Check sheet for the modelled part. Datum: model origin and axes. Units: mm. A direction names the side the tool comes from. Round coordinates to 2 decimals unless told otherwise and drop trailing zeros. Order: outer loops, then holes, each group sorted by start corner. A loop starts at its lowest first (then second) coordinate and runs counter-clockwise, first axis right, second up. Notation, with made-up numbers: (88.5, 67.25) -> (118.5, 67.25) arc R16 ccw to (118.5, 73.25) -> close; hole circle Ø10 at (47, 5). An arc over 180 degrees is marked (long way). Use CSV: the item, a comma, the result in double quotes.
Autodesk Inventor part; units mm, degrees
ref_plane "YZ Plane" through (0, 0, 0) normal (1, 0, 0) x (0, 1, 0)
ref_plane "XZ Plane" through (0, 0, 0) normal (0, 1, 0) x (-1, 0, 0)
ref_plane "XY Plane" through (0, 0, 0) normal (0, 0, 1) x (1, 0, 0)
sketch "Sketch1" plane through (0, 0, 0) normal (0, 1, 0) x (-1, 0, 0)
  circle A0 centre (0, 0) radius 300
  circle A1 centre (0, 0) radius 320
  line L0 (320, 0) -> (300, 0)
  line L1 (-320, 0) -> (-300, 0)
  line L2 (0, 0) -> (-300, 0) construction
  line L3 (0, 300) -> (0, 0) construction
  line L4 (0, 320) -> (0, 300)
  line L5 (-300, 0) -> (-320, 0)
  line L6 (-304, 7) -> (-316, 7)
  line L7 (-316, 7) -> (-313.4522, 0)
  line L8 (-304, 7) -> (-306.5478, 0)
  line L9 (-310, 0) -> (-310, 7) construction
  line L10 (-306.201, 57.7437) -> (-299.2289, 86.9223)
  line L11 (-299.2289, 86.9223) -> (-296.1165, 86.1786)
  line L12 (-296.1165, 86.1786) -> (-303.0886, 57)
  line L13 (-303.0886, 57) -> (-306.201, 57.7437)
  line L14 (-306.201, 57.7437) -> (-296.1165, 86.1786) construction
  line L15 (-299.2289, 86.9223) -> (-303.0886, 57) construction
  circle A2 centre (0, 0) radius 310 construction
  line L16 (-7, -304) -> (0, -306.5478)
  line L17 (-7, -316) -> (0, -313.4522)
  line L18 (-7, -304) -> (-7, -316)
  line L19 (304, -7) -> (306.5478, 0)
  line L20 (316, -7) -> (313.4522, 0)
  line L21 (304, -7) -> (316, -7)
  line L22 (7, 304) -> (0, 306.5478)
  line L23 (7, 316) -> (0, 313.4522)
  line L24 (7, 304) -> (7, 316)
  line L25 (-294.0497, -103.093) -> (-302.6009, -74.3375)
  line L26 (-290.9825, -102.1809) -> (-294.0497, -103.093)
  line L27 (-299.5337, -73.4254) -> (-290.9825, -102.1809)
  line L28 (-302.6009, -74.3375) -> (-299.5337, -73.4254)
  line L29 (-203.108, -236.306) -> (-224.8913, -215.6787)
  line L30 (-200.9078, -233.9825) -> (-203.108, -236.306)
  line L31 (-222.6911, -213.3551) -> (-200.9078, -233.9825)
  line L32 (-224.8913, -215.6787) -> (-222.6911, -213.3551)
  line L33 (-57.7437, -306.201) -> (-86.9223, -299.2289)
  line L34 (-57, -303.0886) -> (-57.7437, -306.201)
  line L35 (-86.1786, -296.1165) -> (-57, -303.0886)
  line L36 (-86.9223, -299.2289) -> (-86.1786, -296.1165)
  line L37 (103.093, -294.0497) -> (74.3375, -302.6009)
  line L38 (102.1809, -290.9825) -> (103.093, -294.0497)
  line L39 (73.4254, -299.5337) -> (102.1809, -290.9825)
  line L40 (74.3375, -302.6009) -> (73.4254, -299.5337)
  line L41 (236.306, -203.108) -> (215.6787, -224.8913)
  line L42 (233.9825, -200.9078) -> (236.306, -203.108)
  line L43 (213.3551, -222.6911) -> (233.9825, -200.9078)
  line L44 (215.6787, -224.8913) -> (213.3551, -222.6911)
  line L45 (306.201, -57.7437) -> (299.2289, -86.9223)
  line L46 (303.0886, -57) -> (306.201, -57.7437)
  line L47 (296.1165, -86.1786) -> (303.0886, -57)
  line L48 (299.2289, -86.9223) -> (296.1165, -86.1786)
  line L49 (294.0497, 103.093) -> (302.6009, 74.3375)
  line L50 (290.9825, 102.1809) -> (294.0497, 103.093)
  line L51 (299.5337, 73.4254) -> (290.9825, 102.1809)
  line L52 (302.6009, 74.3375) -> (299.5337, 73.4254)
  line L53 (203.108, 236.306) -> (224.8913, 215.6787)
  line L54 (200.9078, 233.9825) -> (203.108, 236.306)
  line L55 (222.6911, 213.3551) -> (200.9078, 233.9825)
  line L56 (224.8913, 215.6787) -> (222.6911, 213.3551)
  line L57 (57.7437, 306.201) -> (86.9223, 299.2289)
  line L58 (57, 303.0886) -> (57.7437, 306.201)
  line L59 (86.1786, 296.1165) -> (57, 303.0886)
  line L60 (86.9223, 299.2289) -> (86.1786, 296.1165)
  line L61 (-103.093, 294.0497) -> (-74.3375, 302.6009)
  line L62 (-102.1809, 290.9825) -> (-103.093, 294.0497)
  line L63 (-73.4254, 299.5337) -> (-102.1809, 290.9825)
  line L64 (-74.3375, 302.6009) -> (-73.4254, 299.5337)
  line L65 (-236.306, 203.108) -> (-215.6787, 224.8913)
  line L66 (-233.9825, 200.9078) -> (-236.306, 203.108)
  line L67 (-213.3551, 222.6911) -> (-233.9825, 200.9078)
  line L68 (-215.6787, 224.8913) -> (-213.3551, 222.6911)
  point P0 (310, 0)
  point P1 (-310, 0)
  point P2 (-301.1588, 71.9611)
  point P3 (-59.267, 304.2818)
  point P4 (-304.6448, 57.3718)
  point P5 (-297.6727, 86.5504)
  point P6 (-7, -310)
  point P7 (310, -7)
  point P8 (7, 310)
  point P9 (-292.5161, -102.6369)
  point P10 (-301.0673, -73.8815)
  point P11 (-202.0079, -235.1442)
  point P12 (-223.7912, -214.5169)
  point P13 (-57.3718, -304.6448)
  point P14 (-86.5504, -297.6727)
  point P15 (102.6369, -292.5161)
  point P16 (73.8815, -301.0673)
  point P17 (235.1442, -202.0079)
  point P18 (214.5169, -223.7912)
  point P19 (304.6448, -57.3718)
  point P20 (297.6727, -86.5504)
  point P21 (292.5161, 102.6369)
  point P22 (301.0673, 73.8815)
  point P23 (202.0079, 235.1442)
  point P24 (223.7912, 214.5169)
  point P25 (57.3718, 304.6448)
  point P26 (86.5504, 297.6727)
  point P27 (-102.6369, 292.5161)
  point P28 (-73.8815, 301.0673)
  point P29 (-235.1442, 202.0079)
  point P30 (-214.5169, 223.7912)
  point P31 (-306.5478, 0)
  point P32 (0, 306.5478)
  point P33 (0, 313.4522)
  point P34 (-313.4522, 0)
  dimension "d0" = 600
  dimension "d1" = 640
  dimension "d4" = 90
  dimension "d5" = 7
  dimension "d6" = 70
  dimension "d8" = 12
  dimension "d13" = 3.2
  dimension "d14" = 30
  dimension "d15" = 50
  dimension "d20" = 620
  dimension "d23" = 360
  dimension "d27" = 360
extrude "Extrusion1" add sketch "Sketch1" along normal blind 3 contours A0 L1 L8 L6 L7 A1 L4 | L4 L23 L24 L22
properties part number "R60_CM_CIRCULO"
Q1. Sectioned sample at C-C, the plane x = 49.5. Enter the section's corners in (y, z).
Result sheet:
outline,"(0, 295.89) -> (3, 295.89) -> (3, 316.15) -> (0, 316.15) -> close"
Q2. Mould release check, pull along Z, two halves, no side actions. Record for faces 1 (the face through (228.75, 1.48, 223.77)), 2 (the face through (218, 3, 208)), 3 (the face through (302.764, 1.479, 72.129)), 4 (the face through (214.45, 1.48, 209.79)): pulls with the +Z half, pulls with the -Z half, needs draft (parallel to the pull), parting line crosses it, or undercut.
Result sheet:
face 1,"pulls with the +Z half"
face 2,"needs draft"
face 3,"undercut"
face 4,"pulls with the -Z half"
Q3. Access from +Z, -Z, +X, -X, +Y, -Y to the whole of each face (thin tool, end or side, straight path). Record for faces 5 (the face through (218, 0, 208)), 6 (the face through (223.524, 1.479, 211.952)).
Result sheet:
face 5,"+Z, -Z, +X, -X, -Y"
face 6,"+Y, -Y"
Q4. Sectioned sample at B-B, the plane z = 40.5. Enter the section's corners in (x, y), then the cut area to 3 significant figures.
Result sheet:
outline,"(297.25, 0) -> (317.43, 0) -> (317.43, 3) -> (297.25, 3) -> close"
area,"60.5 mm^2"
Q5. Go/stop test with a flat-tipped pin: pin 1 (8 mm diameter, centred on x = 219.5, z = 243, fed in from +Y). Record where the tip stops, or that it passes through.
Result sheet:
pin 1,"passes through"
Q6. Scan lines: L1, parallel to X at y = 0.3, z = 210; L2, parallel to Z at x = 217.5, y = 1.2; L3, parallel to X at y = 1.15, z = 192.5. Record each from-to range of solid material in increasing order.
Result sheet:
L1,"x = 214.24 to 225.37, 229.78 to 241.45"
L2,"z = 206.62 to 218.31, 222.97 to 234.72"
L3,"x = 230.1 to 255.62"
Q7. Sectioned sample at A-A, the plane y = 0.9. Enter the section's corners in (x, z).
Result sheet:
outline,"(-7, 304) -> (0, 306.55) -> (0, 300) arc R300 cw to (300, 0) -> (306.55, 0) -> (304, 7) -> (316, 7) -> (313.45, 0) -> (320, 0) arc R320 ccw to (0, 320) -> (0, 313.45) -> (-7, 316) -> close; hole (73.43, 299.53) -> (102.18, 290.98) -> (103.09, 294.05) -> (74.34, 302.6) -> close; hole (213.36, 222.69) -> (233.98, 200.91) -> (236.31, 203.11) -> (215.68, 224.89) -> close; hole (296.12, 86.18) -> (303.09, 57) -> (306.2, 57.74) -> (299.23, 86.92) -> close"
